```python
from build123d import *

# Parameters (mm, degrees)
F1_DEPTH = 63.5
F0_W     = 23.975106
F0_H     = 19.05
F2_DEPTH = 25.4
F3_DEPTH = 12.7
F5_R     = 6.35


with BuildPart() as f1:
    # F0 (on Front) → F1 (new body, symmetric)
    with BuildSketch(Plane.XZ):
        Polygon((-41.275, 9.525), (-41.275, -9.525), (41.275, -9.525), (41.275, 9.525), (22.225, 9.525), align=None)
    extrude(amount=F1_DEPTH, both=True)

    # F0 (on Front) → F2 (join, symmetric)
    with BuildSketch(Plane.XZ):
        with BuildLine():
            Line((22.225, 9.525), (41.275, 9.525))
            Line((41.275, 9.525), (41.275, 27.0002))
            ThreePointArc((41.275, 27.0002), (45.92468, 38.22552), (57.15, 42.8752))
            Line((57.15, 42.8752), (60.325, 42.8752))
            Line((60.325, 42.8752), (60.325, 61.9252))
            Line((60.325, 61.9252), (57.15, 61.9252))
            ThreePointArc((57.15, 61.9252), (32.454296, 51.695904), (22.225, 27.0002))
            Line((22.225, 27.0002), (22.225, 9.525))
        make_face()
        with Locations((72.312553, 52.4002)):
            Rectangle(F0_W, F0_H)
    extrude(amount=F2_DEPTH, both=True)

    # F0 (on Front) → F3 (join, symmetric)
    with BuildSketch(Plane.XZ):
        with BuildLine():
            add(Edge.make_bspline(
                [(-41.275, 9.525), (-18.111696, 56.123264), (21.593637, 63.694689), (57.15, 61.9252)],
                knots=[0, 0, 0, 0, 111.504536, 111.504536, 111.504536, 111.504536], degree=3))
            Line((-41.275, 9.525), (22.225, 9.525))
            Line((22.225, 9.525), (22.225, 27.0002))
            ThreePointArc((22.225, 27.0002), (32.454296, 51.695904), (57.15, 61.9252))
        make_face()
    extrude(amount=F3_DEPTH, both=True)

    # F0 (on Front) → F4 (revolve)
    with BuildSketch(Plane.XZ):
        Polygon((111.125, 66.675), (85.725, 66.675), (85.725, 52.3875), (85.725, 38.1), (111.125, 38.1), align=None)
    revolve(axis=Axis((85.725, 0, 61.228485), (0, 0, 1)))

    # F5
    f5_edges = [f1.edges().sort_by_distance(p)[0] for p in [
        (41.275, -63.5, 0),
        (-41.275, -63.5, 0),
        (41.275, 63.5, 0),
        (-41.275, 63.5, 0),
    ]]
    fillet(f5_edges, radius=F5_R)


solid = f1.part
```
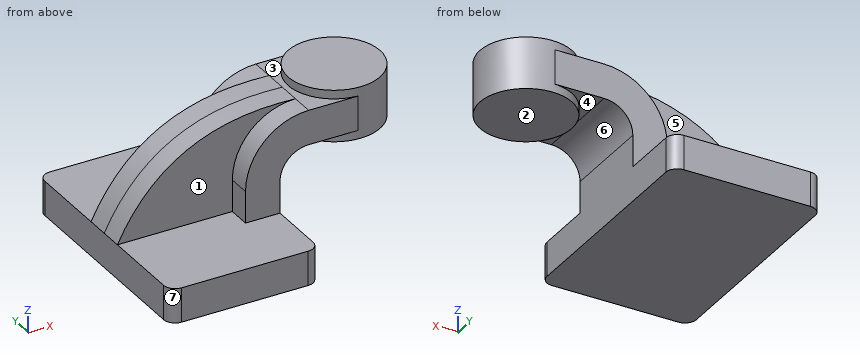
Can you work these out from the model? Positions are in its coordinate system, mm. Face numbers are marked on the shaded views. A direction names the side the tool comes from. Coordinates: 2 decimals unless noted, no trailing zeros. Loops run counter-clockwise (first coordinate to the right, second up) from the corner with the lowest first, then second, coordinate; pieces in that order, holes last.
1) Imagine slicing it at A-A on y = 28. List the corners of the cut face in (x, z) for me (3 decimals).
2) For pin 1 (4 mm diameter, centred on x = 23, y = -45, fed in from +Z) (3 decimals); pin 2 (4 mm diameter, centred on x = 29.5, z = 53.5, fed in from +Y); pin 3 (18.5 mm diameter, centred on y = 26.5, z = 15, fed in from +X) (3 decimals), each with a flat end and sliding along its axis, tell me the tip position at first contact or that it passes through.
3) Which directions (+Z, -Z, +X, -X, +Y, -Y) give clear straight access to the entire face, cutting with the end or side of a thin tool? Please do the marked faces 1, 2 and 3.
4) I need wall thicknesses on probe 1 along Y at (x, z) = (21.5, 58); probe 2 along X at (y, z) = (-19, -2) (3 decimals); probe 3 along X at (y, z) = (19, 23) (3 decimals). Which ranges of each line are inside material? Lowest first, please.
5) Imagine slicing it at B-B on x = 91. List the corners of the cut face in (y, z) for me (3 decimals).
6) Thinking about a two-plate mould opening in X: for the marked faces 4, 5, 6 and 7, which applies, pulls with the +X half, pulls with the -X half, needs draft (parallel to the pull), parting line crosses it, or undercut?
Completed:
1. outline: (-41.275, -9.525) - (41.275, -9.525) - (41.275, 9.525) - (-41.275, 9.525) - close
2. pin 1: stops at z = 9.525
2. pin 2: stops at y = 12.7
2. pin 3: stops at x = 41.275
3. face 1: +Z, -X, -Y
3. face 2: -Z, +X, +Y, -Y
3. face 3: +Z
4. probe 1: y = -12.7 to 12.7
4. probe 2: x = -41.275 to 41.275
4. probe 3: x = 22.225 to 41.275
5. outline: (-24.846, 38.1) - (24.846, 38.1) - (24.846, 66.675) - (-24.846, 66.675) - close
6. face 4: undercut
6. face 5: needs draft
6. face 6: undercut
6. face 7: pulls with the -X half
